Here's how the part is built. I have some questions about the finished solid (model axes, mm). Face numbers are marked on the shaded views. Coordinates: 2 decimals unless noted, no trailing zeros. Write each loop counter-clockwise with the first axis right and the second up, starting at its lowest first coordinate (ties: lowest second). Pieces come first, ordered by that corner, then holes. Notation, with made-up numbers: (-14, -33) -> (20, -33) arc R13 ccw to (20, -27) -> close; hole circle Ø6 at (23.5, 53.5). An arc over 180 degrees is marked (long way). Use a Markdown table: item, result. Add a question column.
Item 1: Imagine slicing it at A-A, the plane x = 54.5. Write out the boundary of the cut face in (y, z).
Item 2: Imagine slicing it at C-C, the plane z = -58.5. Write out the boundary of the cut face in (x, y), and give its area (4 significant figures).
Item 3: Imagine slicing it at D-D, the plane x = 28.5. Write out the boundary of the cut face in (y, z), and give its area (3 significant figures).
Item 4: Imagine slicing it at B-B, the plane z = -94. Write out the boundary of the cut face in (x, y), and give its area (3 significant figures).
Item 5: Will these pins go through, and if not, where does the flat tip stop? pin 1 Ø12 at (x, z) = (113, -42.5) entering from +Y; pin 2 Ø1.5 at (x, y) = (110, 6.5) entering from +Z; pin 3 Ø1.2 at (x, y) = (49.5, 7) entering from -Z.
Item 6: If we mould it in two halves opening along X, with no side actions, what happens to the marked faces 1 and 2? For each: pulls with the +X half, pulls with the -X half, needs draft (parallel to the pull), parting line crosses it, or undercut.
Item 7: If I drill on line 1 along Z through (x, y) = (56, 3.5); line 2 along X through (y, z) = (1.75, -76); line 3 along X through (y, z) = (2, -17.3), over which ranges is the centre line in solid material (lowest first)? Write a range as from..to.
```python
from build123d import *

# Parameters (mm, degrees)
SKETCH1_W           = 126
SKETCH1_H           = 126
BOSS_EXTRUDE1_DEPTH = 5
SKETCH3_R           = 12.5
BOSS_EXTRUDE2_DEPTH = 7.5
SKETCH4_R           = 3.45
CUT_EXTRUDE1_DEPTH  = 11.5
SKETCH6_R           = 3
CUT_EXTRUDE2_DEPTH  = 179.628805068
CHAMFER1_SIZE       = 10
CHAMFER1_SIZE_2     = 7.26542528
SKETCH7_W           = 8
SKETCH7_H           = 77.91635632
BOSS_EXTRUDE3_DEPTH = 3
SKETCH8_R           = 3
CUT_EXTRUDE3_DEPTH  = 179.370401132
SKETCH9_R           = 3.45
CUT_EXTRUDE4_DEPTH  = 7
SKETCH10_W          = 85.5
SKETCH10_H          = 55.5
SKETCH10_H_2        = 37.1
SKETCH10_W_2        = 73.5
SKETCH10_H_3        = 19.1
SKETCH10_W_3        = 36.75
SKETCH10_H_4        = 9.55
BOSS_EXTRUDE5_DEPTH = 1.5
SKETCH12_W          = 79.5
SKETCH12_H          = 49.5
BOSS_EXTRUDE6_DEPTH = 1.5
SKETCH13_W          = 79.5
SKETCH13_H          = 31.1
BOSS_EXTRUDE7_DEPTH = 1.5
SKETCH14_W          = 24.8
SKETCH14_H          = 35
CUT_EXTRUDE5_DEPTH  = 179.370401132
SKETCH15_W          = 12.8
SKETCH15_H          = 19.5
CUT_EXTRUDE6_DEPTH  = 179.370401132
SKETCH16_R          = 3
CUT_EXTRUDE7_DEPTH  = 179.370401132


with BuildPart() as part:
    # Sketch1 → Boss-Extrude1 (new body)
    with BuildSketch(Plane(origin=(0, 0, 0), x_dir=(1, 0, 0), z_dir=(0, 1, 0))):
        with Locations((63, 63)):
            Rectangle(SKETCH1_W, SKETCH1_H)
    extrude(amount=BOSS_EXTRUDE1_DEPTH)

    # Sketch3 → Boss-Extrude2 (add)
    with BuildSketch(Plane(origin=(0, 5, 0), x_dir=(1, 0, 0), z_dir=(0, 1, 0))):
        with Locations(Location((108.6, 108.6, 0), (0, 0, 90))):
            Circle(SKETCH3_R)
    extrude(amount=BOSS_EXTRUDE2_DEPTH)

    # Sketch4 → Cut-Extrude1 (cut)
    with BuildSketch(Plane.XZ):
        with Locations(Location((108.6, -108.6, 0), (0, 0, 270))):
            Circle(SKETCH4_R)
    extrude(amount=-CUT_EXTRUDE1_DEPTH, mode=Mode.SUBTRACT)

    # Sketch6 → Cut-Extrude2 (cut, through all)
    with BuildSketch(Plane(origin=(0, 12.5, 0), x_dir=(1, 0, 0), z_dir=(0, 1, 0))):
        with Locations(Location((108.6, 108.6, 0), (0, 0, 270))):
            Circle(SKETCH6_R)
    extrude(amount=-CUT_EXTRUDE2_DEPTH, mode=Mode.SUBTRACT)

    # Chamfer1
    # the kernel refuses this chamfer: 10, 7.26542528 mm, written as the material it takes off along each edge
    with BuildSketch(Plane(origin=(108.6, 12.5, -108.6), x_dir=(0, 0, -1), z_dir=(1, 0, 0))) as chamfer1_piece_1_section:
        Polygon((12.5, -CHAMFER1_SIZE), (12.5 - CHAMFER1_SIZE_2, 0), (12.5, 0), align=None)
    chamfer1_piece_1 = revolve(axis=Axis((108.6, 12.5, -108.6), (0, 1, 0)), mode=Mode.PRIVATE)
    chamfer1_piece_1 = split(chamfer1_piece_1, bisect_by=Plane(origin=(108.6, 5, -100.650989912), z_dir=(0, 1, 0)), keep=Keep.TOP, mode=Mode.PRIVATE)
    add(chamfer1_piece_1, mode=Mode.SUBTRACT)

    # Sketch7 → Boss-Extrude3 (add)
    with BuildSketch(Plane(origin=(0, 5, 0), x_dir=(1, 0, 0), z_dir=(0, 1, 0))):
        with Locations((108.6, 48.95817816)):
            Rectangle(SKETCH7_W, SKETCH7_H)
    extrude(amount=BOSS_EXTRUDE3_DEPTH)

    # Sketch8 → Cut-Extrude3 (cut, through all)
    with BuildSketch(Plane(origin=(0, 8, 0), x_dir=(1, 0, 0), z_dir=(0, 1, 0))):
        with Locations(Location((108.6, 15, 0), (0, 0, 270))):
            Circle(SKETCH8_R)
        with Locations(Location((108.6, 31.974801407, 0), (0, 0, 270))):
            Circle(SKETCH8_R)
        with Locations(Location((108.6, 48.949602814, 0), (0, 0, 270))):
            Circle(SKETCH8_R)
        with Locations(Location((108.6, 65.924404221, 0), (0, 0, 270))):
            Circle(SKETCH8_R)
        with Locations(Location((108.6, 82.899205628, 0), (0, 0, 270))):
            Circle(SKETCH8_R)
    extrude(amount=-CUT_EXTRUDE3_DEPTH, mode=Mode.SUBTRACT)

    # Sketch9 → Cut-Extrude4 (cut)
    with BuildSketch(Plane.XZ):
        with Locations(Location((108.6, -82.899205628, 0), (0, 0, 270))):
            Circle(SKETCH9_R)
        with Locations(Location((108.6, -65.924404221, 0), (0, 0, 270))):
            Circle(SKETCH9_R)
        with Locations(Location((108.6, -48.949602814, 0), (0, 0, 270))):
            Circle(SKETCH9_R)
        with Locations(Location((108.6, -15, 0), (0, 0, 270))):
            Circle(SKETCH9_R)
        with Locations(Location((108.6, -31.974801407, 0), (0, 0, 270))):
            Circle(SKETCH9_R)
    extrude(amount=-CUT_EXTRUDE4_DEPTH, mode=Mode.SUBTRACT)

    # Sketch10 → Boss-Extrude5 (add)
    # profile 1 of 6: a face of its own
    with BuildSketch(Plane(origin=(0, 5, 0), x_dir=(1, 0, 0), z_dir=(0, 1, 0))):
        with Locations((48.95817816, 80.85)):
            Rectangle(SKETCH10_W, SKETCH10_H)
    # profile 2 of 6: a face of its own
    with BuildSketch(Plane(origin=(0, 5, 0), x_dir=(1, 0, 0), z_dir=(0, 1, 0))):
        with Locations((48.95817816, 28.55)):
            Rectangle(SKETCH10_W, SKETCH10_H_2)
        with Locations((48.95817816, 31.55)):
            Rectangle(SKETCH10_W_2, SKETCH10_H_3, mode=Mode.SUBTRACT)
    # profile 3 of 6: a face of its own
    with BuildSketch(Plane(origin=(0, 5, 0), x_dir=(1, 0, 0), z_dir=(0, 1, 0))):
        with Locations((30.58317816, 26.775)):
            Rectangle(SKETCH10_W_3, SKETCH10_H_4)
    # profile 4 of 6: a face of its own
    with BuildSketch(Plane(origin=(0, 5, 0), x_dir=(1, 0, 0), z_dir=(0, 1, 0))):
        with Locations((30.58317816, 36.325)):
            Rectangle(SKETCH10_W_3, SKETCH10_H_4)
    # profile 5 of 6: a face of its own
    with BuildSketch(Plane(origin=(0, 5, 0), x_dir=(1, 0, 0), z_dir=(0, 1, 0))):
        with Locations((67.33317816, 36.325)):
            Rectangle(SKETCH10_W_3, SKETCH10_H_4)
    # profile 6 of 6: a face of its own
    with BuildSketch(Plane(origin=(0, 5, 0), x_dir=(1, 0, 0), z_dir=(0, 1, 0))):
        with Locations((67.33317816, 26.775)):
            Rectangle(SKETCH10_W_3, SKETCH10_H_4)
    extrude(amount=BOSS_EXTRUDE5_DEPTH)

    # Sketch12 → Boss-Extrude6 (add)
    with BuildSketch(Plane(origin=(0, 6.5, 0), x_dir=(1, 0, 0), z_dir=(0, 1, 0))):
        with Locations((48.95817816, 80.85)):
            Rectangle(SKETCH12_W, SKETCH12_H)
    extrude(amount=BOSS_EXTRUDE6_DEPTH)

    # Sketch13 → Boss-Extrude7 (add)
    with BuildSketch(Plane(origin=(0, 6.5, 0), x_dir=(1, 0, 0), z_dir=(0, 1, 0))):
        with Locations((48.95817816, 28.55)):
            Rectangle(SKETCH13_W, SKETCH13_H)
    extrude(amount=BOSS_EXTRUDE7_DEPTH)

    # Sketch14 → Cut-Extrude5 (cut, through all)
    with BuildSketch(Plane(origin=(0, 8, 0), x_dir=(1, 0, 0), z_dir=(0, 1, 0))):
        with Locations((48.95817816, 80.85)):
            Rectangle(SKETCH14_W, SKETCH14_H)
    extrude(amount=-CUT_EXTRUDE5_DEPTH, mode=Mode.SUBTRACT)

    # Sketch15 → Cut-Extrude6 (cut, through all)
    with BuildSketch(Plane(origin=(0, 8, 0), x_dir=(1, 0, 0), z_dir=(0, 1, 0))):
        with Locations((38.862130436, 31.35)):
            Rectangle(SKETCH15_W, SKETCH15_H)
        with Locations((18.262130436, 31.35)):
            Rectangle(SKETCH15_W, SKETCH15_H)
        with Locations((59.462130436, 31.35)):
            Rectangle(SKETCH15_W, SKETCH15_H)
        with Locations((80.062130436, 31.35)):
            Rectangle(SKETCH15_W, SKETCH15_H)
    extrude(amount=-CUT_EXTRUDE6_DEPTH, mode=Mode.SUBTRACT)

    # Sketch16 → Cut-Extrude7 (cut, through all)
    with BuildSketch(Plane(origin=(0, 8, 0), x_dir=(1, 0, 0), z_dir=(0, 1, 0))):
        with Locations(Location((18.262130436, 17.3, 0), (0, 0, 270))):
            Circle(SKETCH16_R)
        with Locations(Location((38.862130436, 16.84840868, 0), (0, 0, 270))):
            Circle(SKETCH16_R)
        with Locations(Location((59.462130436, 17.3, 0), (0, 0, 270))):
            Circle(SKETCH16_R)
        with Locations(Location((80.062130436, 17.3, 0), (0, 0, 270))):
            Circle(SKETCH16_R)
    extrude(amount=-CUT_EXTRUDE7_DEPTH, mode=Mode.SUBTRACT)


solid = part.part
```
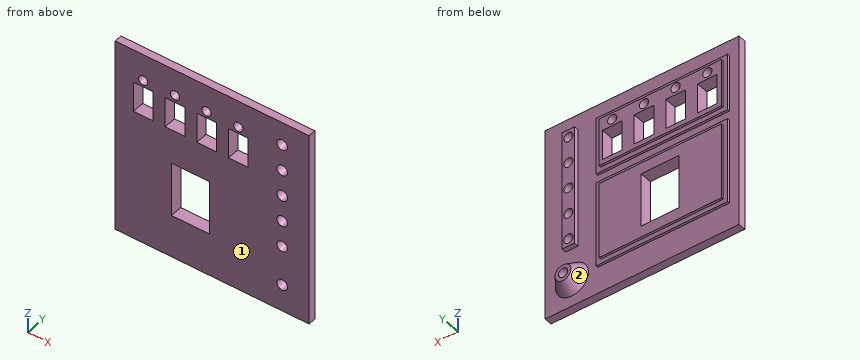
Ans:
| question | item | result |
|---|---|---|
| 1 | outline | (0, -126) -> (5, -126) -> (5, -108.6) -> (6.5, -108.6) -> (6.5, -105.6) -> (8, -105.6) -> (8, -98.35) -> (0, -98.35) -> close; (0, -63.35) -> (8, -63.35) -> (8, -56.1) -> (6.5, -56.1) -> (6.5, -53.1) -> (5, -53.1) -> (5, -47.1) -> (6.5, -47.1) -> (6.5, -44.1) -> (8, -44.1) -> (8, -41.1) -> (0, -41.1) -> close; (0, -21.6) -> (8, -21.6) -> (8, -13) -> (6.5, -13) -> (6.5, -10) -> (5, -10) -> (5, 0) -> (0, 0) -> close |
| 2 | outline | (0, 0) -> (126, 0) -> (126, 5) -> (112.6, 5) -> (112.6, 8) -> (104.6, 8) -> (104.6, 5) -> (91.71, 5) -> (91.71, 6.5) -> (88.71, 6.5) -> (88.71, 8) -> (9.21, 8) -> (9.21, 6.5) -> (6.21, 6.5) -> (6.21, 5) -> (0, 5) -> close |
| 2 | area | 901.5 mm^2 |
| 3 | outline | (0, -126) -> (5, -126) -> (5, -108.6) -> (6.5, -108.6) -> (6.5, -105.6) -> (8, -105.6) -> (8, -56.1) -> (6.5, -56.1) -> (6.5, -53.1) -> (5, -53.1) -> (5, -47.1) -> (6.5, -47.1) -> (6.5, -44.1) -> (8, -44.1) -> (8, -13) -> (6.5, -13) -> (6.5, -10) -> (5, -10) -> (5, 0) -> (0, 0) -> close |
| 3 | area | 890 mm^2 |
| 4 | outline | (0, 0) -> (36.56, 0) -> (36.56, 8) -> (9.21, 8) -> (9.21, 6.5) -> (6.21, 6.5) -> (6.21, 5) -> (0, 5) -> close; (61.36, 0) -> (126, 0) -> (126, 5) -> (91.71, 5) -> (91.71, 6.5) -> (88.71, 6.5) -> (88.71, 8) -> (61.36, 8) -> close |
| 4 | area | 679 mm^2 |
| 5 | pin 1 | stops at y = 8 |
| 5 | pin 2 | stops at z = -10 |
| 5 | pin 3 | stops at z = -108.6 |
| 6 | face 1 | needs draft |
| 6 | face 2 | undercut |
| 7 | line 1 | z = -126..-98.35, -63.35..-41.1, -21.6..0 |
| 7 | line 2 | x = 0..36.56, 61.36..126 |
| 7 | line 3 | x = 0..15.26, 21.26..35.9, 41.83..56.46, 62.46..77.06, 83.06..106.03, 111.17..126 |
